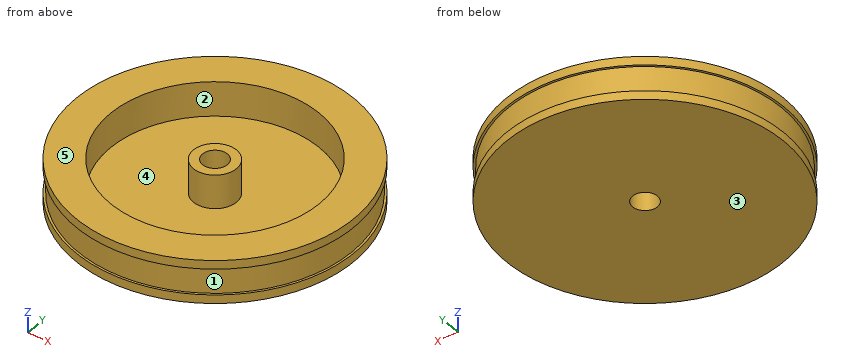
from build123d import *

# Parameters (mm, degrees)
F2_R     = 5
F3_DEPTH = 7.8
F4_R     = 2.88696
F5_DEPTH = 25


with BuildPart() as f1:
    # F0 (on Front) → F1 (revolve)
    with BuildSketch(Plane.XZ):
        Polygon((-32.2, 0), (0, 0), (0, 2), (-24.2, 2), (-24.2, 10), (-32.2, 10), (-32.2, 8), (-31.7, 8), (-31.7, 2), (-32.2, 2), align=None)
    revolve(axis=Axis((0, 0, 1), (0, 0, -1)))

    # F2 (on face) → F3 (join)
    with BuildSketch(Plane.XY.offset(2)):
        Circle(F2_R)
    extrude(amount=F3_DEPTH)

    # F4 (on face) → F5 (cut)
    with BuildSketch(Plane.XY.offset(9.8)):
        Circle(F4_R)
    extrude(amount=-F5_DEPTH, mode=Mode.SUBTRACT)


solid = f1.part
The listing builds one solid part. Answer for the finished solid, in the listing's coordinates (mm). Face numbers are marked on the shaded views. A direction names the side the tool comes from. Coordinates: 2 decimals unless noted, no trailing zeros. Order: outer loops, then holes, each group sorted by start corner. A loop starts at its lowest first (then second) coordinate and runs counter-clockwise, first axis right, second up.
Q1. For a pull along X with two mould halves and no side action, classify the marked faces 1, 2 and 3 as pulls with the +X half, pulls with the -X half, needs draft (parallel to the pull), parting line crosses it, or undercut.
Q2. Which of the six approach directions +Z, -Z, +X, -X, +Y, -Y give full straight-line access (tool end or side, diameter ignored) to the marked faces 4 and 5?
Q3. Given P1, Ø3, axis at x = -0.5, y = -2, coming from the +Z side; P2, Ø1, axis at x = -1, z = 2, coming from the -Y side; P3, Ø6, axis at x = -10.5, z = 5.5, coming from the +Y side, each flat-ended and moving along its own axis, determine where each tip first touches the part or whether it passes through.
Q4. A cutting plane is placed at D-D, the plane y = -15. Write down the section's boundary in (x, z), and give its area (3 significant figures).
Q5. A cutting plane is placed at A-A, the plane x = 0. Write down the section's boundary in (y, z).
Q6. Consider line 1 (Y direction, x = 0, z = 7.5); line 2 (X direction, y = -2, z = 5); line 3 (X direction, y = -3.5, z = 9). Determine where each line is inside the solid, lowest interval first.
Q7. A cutting plane is placed at C-C, the plane z = 6.25. Write down the section's boundary in (x, y).
Answers follow:
1. face 1: parting line crosses it
1. face 2: undercut
1. face 3: needs draft
2. face 4: +Z
2. face 5: +Z, +X, -X, +Y, -Y
3. P1: stops at z = 9.8
3. P2: stops at y = -32.2
3. P3: stops at y = 30.96
4. outline: (-28.49, 0) - (28.49, 0) - (28.49, 2) - (27.93, 2) - (27.93, 8) - (28.49, 8) - (28.49, 10) - (18.99, 10) - (18.99, 2) - (-18.99, 2) - (-18.99, 10) - (-28.49, 10) - (-28.49, 8) - (-27.93, 8) - (-27.93, 2) - (-28.49, 2) - close
4. area: 259 mm2
5. outline: (-32.2, 0) - (-2.89, 0) - (-2.89, 9.8) - (-5, 9.8) - (-5, 2) - (-24.2, 2) - (-24.2, 10) - (-32.2, 10) - (-32.2, 8) - (-31.7, 8) - (-31.7, 2) - (-32.2, 2) - close; (2.89, 0) - (32.2, 0) - (32.2, 2) - (31.7, 2) - (31.7, 8) - (32.2, 8) - (32.2, 10) - (24.2, 10) - (24.2, 2) - (5, 2) - (5, 9.8) - (2.89, 9.8) - close
6. line 1: y = -31.7 to -24.2, -5 to -2.89, 2.89 to 5, 24.2 to 31.7
6. line 2: x = -31.64 to -24.12, -4.58 to -2.08, 2.08 to 4.58, 24.12 to 31.64
6. line 3: x = -32.01 to -23.95, -3.57 to 3.57, 23.95 to 32.01
7. outline: circle Ø63.4 at (0, 0); circle Ø10 at (0, 0); hole circle Ø48.4 at (0, 0); hole circle Ø5.77 at (0, 0)
